Answer from the drawing. Dimensions are ordinates in mm from the lowest x, y and z of the part. A direction names the side the tool comes from. Coordinates: 2 decimals unless noted, no trailing zeros. Order: outer loops, then holes, each group sorted by start corner. A loop starts at its lowest first (then second) coordinate and runs counter-clockwise, first axis right, second up. Notation, with made-up numbers: (-31.75, 64.25) -> (-24.75, 64.25) arc R18 ccw to (-24.75, 83.25) -> close; hole circle Ø9 at (8.25, -17.75). An arc over 180 degrees is marked (long way). Answer as a JSON object with one key per item and string values. Group by question number.
1) Given pin 1 (6.5 mm diameter, centred on x = 6, z = 32.5, fed in from -Y); pin 2 (8 mm diameter, centred on y = 13, z = 19.5, fed in from -X); pin 3 (1.5 mm diameter, centred on x = 9, y = 11.5, fed in from -Z), each flat-ended and moving along its own axis, determine where each tip first touches the part or whether it passes through.
2) Determine the mould class of the marked faces 4, 5, 6 and 7 for opening direction Y: released by +Y, released by -Y, zero draft, split by the parting line, or undercut.
3) Section A-A on z = 16.5 is taken. Determine the outline of the cut face in (x, y).
4) Section B-B on x = 14 is taken. Determine the outline of the cut face in (y, z).
5) A tool of negligible diameter and unlimited length cuts with its end or side. For the marked faces 1, 2 and 3, from which of +Z, -Z, +X, -X, +Y, -Y can it reach the whole face along a straight path? Write none if from no direction.
6) Consider L1, parallel to X at y = 14, z = 7.5; L2, parallel to Z at x = 14.25, y = 4. Determine where each line is inside the solid, lowest interval first.
7) Section C-C on z = 8 is taken. Determine the outline of the cut face in (x, y).
8) Section D-D on y = 23.5 is taken. Determine the outline of the cut face in (x, z).
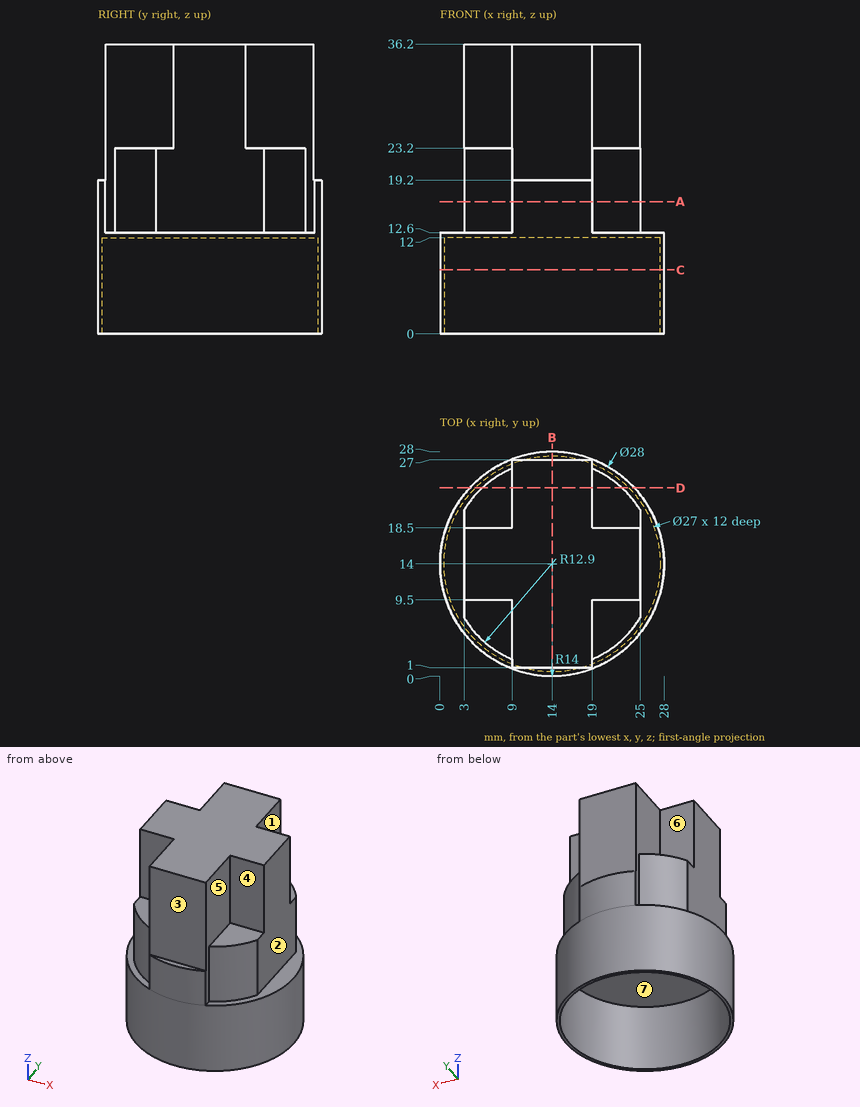
Worked answers:
{
 "1": {"pin 1": "stops at y = 1", "pin 2": "stops at x = 3", "pin 3": "stops at z = 12"},
 "2": {"face 4": "released by -Y", "face 5": "zero draft", "face 6": "released by +Y", "face 7": "undercut"},
 "3": {"outline": "(3, 7.26) arc R12.9 ccw to (9, 2.11) -> (9, 0.92) arc R14 ccw to (19, 0.92) -> (19, 2.11) arc R12.9 ccw to (25, 7.26) -> (25, 20.74) arc R12.9 ccw to (19, 25.89) -> (19, 27.08) arc R14 ccw to (9, 27.08) -> (9, 25.89) arc R12.9 ccw to (3, 20.74) -> close"},
 "4": {"outline": "(0, 0) -> (0.5, 0) -> (0.5, 12) -> (27.5, 12) -> (27.5, 0) -> (28, 0) -> (28, 19.2) -> (27, 19.2) -> (27, 36.2) -> (1, 36.2) -> (1, 19.2) -> (0, 19.2) -> close"},
 "5": {"face 1": "+Z, +X, +Y", "face 2": "+Z, +X, +Y, -Y", "face 3": "+Z, +X, -X, -Y"},
 "6": {"L1": "x = 0 to 0.5, 27.5 to 28", "L2": "z = 12 to 36.2"},
 "7": {"outline": "circle Ø28 at (14, 14); hole circle Ø27 at (14, 14)"},
 "8": {"outline": "(3.72, 0) -> (4.41, 0) -> (4.41, 12) -> (23.59, 12) -> (23.59, 0) -> (24.28, 0) -> (24.28, 12.6) -> (22.73, 12.6) -> (22.73, 23.2) -> (19, 23.2) -> (19, 36.2) -> (9, 36.2) -> (9, 23.2) -> (5.27, 23.2) -> (5.27, 12.6) -> (3.72, 12.6) -> close"}
}
